from build123d import *

# Parameters (mm, degrees)
BOSS_EXTRUDE1_DEPTH = 10
SKETCH2_R           = 2.5
BOSS_EXTRUDE2_DEPTH = 35


with BuildPart() as part:
    # Sketch1 → Boss-Extrude1 (new body)
    with BuildSketch(Plane(origin=(0, 0, 0), x_dir=(0, 0, -1), z_dir=(1, 0, 0))):
        with BuildLine():
            Line((0, 7.5), (20.5, 7.5))
            Line((20.5, 7.5), (20.5, -7.5))
            Line((20.5, -7.5), (0, -7.5))
            ThreePointArc((0, -7.5), (-7.5, 0), (0, 7.5))
        make_face()
        Polygon((5.05, 0), (2.525, 4.373428289), (-2.525, 4.373428289), (-5.05, 0), (-2.525, -4.373428289), (2.525, -4.373428289), align=None, mode=Mode.SUBTRACT)
    extrude(amount=BOSS_EXTRUDE1_DEPTH)

    # Sketch2 → Boss-Extrude2 (add)
    with BuildSketch(Plane(origin=(10, 0, 0), x_dir=(0, 0, -1), z_dir=(1, 0, 0))):
        with Locations((17.956042915, 0)):
            Circle(SKETCH2_R)
    extrude(amount=BOSS_EXTRUDE2_DEPTH)


solid = part.part
Build history of the part. All positions in model axes, mm. A direction names the side the tool comes from. Give positions to 0.01 mm unless a question says otherwise; leave off trailing zeros. Loops run counter-clockwise (first coordinate to the right, second up) from the corner with the lowest first, then second, coordinate; pieces in that order, holes last. Notation, with made-up numbers: (37.25, 26) - (73.25, 26) arc R12 cw to (73.25, 34) - close; hole circle Ø3 at (63.25, 72.5). An arc over 180 degrees is marked (long way). Write item = value, one per line. Start each with the question number.
1) Drop flat-ended pins along their axis: pin 1 Ø8 at (x, z) = (17, -10.5) entering from -Y; pin 2 Ø2 at (x, z) = (5, 3) entering from +Y; pin 3 Ø4 at (y, z) = (-4.5, -6.5) entering from +X; pin 4 Ø1.5 at (x, y) = (27.5, -1) entering from +Z. Give the stop position or say it passes through.
2) Band-saw the part on B-B on x = 7. Give the cut face in (y, z) (3 decimals).
3) Probe probe 1 along X at (y, z) = (3.75, -4.25); probe 2 along Z at (x, y) = (4.5, -0.75); probe 3 along Y at (x, z) = (39, -17.25). List the from-to ranges inside material, lowest first. Write a range as from..to.
4) Band-saw the part on C-C on x = 25. Give the cut face in (y, z).
5) Pull direction Y, two halves, no side cores. Call faces 4 (the flat face through (5, -4.373, 0)), 5 (the flat face through (10, 0, -7)), 6 (the flat face through (5, 4.373, 0)), 7 (the flat face through (5, -7.5, -10)): +Y half, -Y half, draft (parallel to the pull), parting line (faces both ways), or undercut.
6) Band-saw the part on D-D on y = -6.5. Give the cut face in (x, z).
7) Band-saw the part on A-A on y = 2. Give the cut face in (x, z), plus the area to 3 significant figures.
8) Tool access for faces 1 (the flat face through (4.93, 2.156, -3.805)), 2 (the cylindrical face through (27.26, 0.75, -20.34)), 3 (the flat face through (0, 0, -10)): list every direction of +Z, -Z, +X, -X, +Y, -Y with a clear straight run to the whole face (end or side of a thin tool).
Final values:
q1.pin_1 = through
q1.pin_2 = 7.23
q1.pin_3 = 10
q1.pin_4 = -15.47
q2.outline = (-7.5, -20.5) - (7.5, -20.5) - (7.5, 0) arc R7.5 ccw to (-7.5, 0) - close; hole (-4.373, -2.525) - (0, -5.05) - (4.373, -2.525) - (4.373, 2.525) - (0, 5.05) - (-4.373, 2.525) - close
q3.probe_1 = 0..10
q3.probe_2 = -20.5..-4.62, 4.62..7.46
q3.probe_3 = -2.4..2.4
q4.outline = circle Ø5 at (0, -17.96)
q5.face_4 = undercut
q5.face_5 = draft
q5.face_6 = undercut
q5.face_7 = -Y half
q6.outline = (0, -20.5) - (10, -20.5) - (10, 3.74) - (0, 3.74) - close
q7.outline = (0, -20.5) - (10, -20.5) - (10, -19.46) - (45, -19.46) - (45, -16.46) - (10, -16.46) - (10, -3.9) - (0, -3.9) - close; (0, 3.9) - (10, 3.9) - (10, 7.23) - (0, 7.23) - close
q7.area = 304 mm²
q8.face_1 = +X, -X
q8.face_2 = +X
q8.face_3 = +Z, -Z, -X, +Y, -Y
